from build123d import *

# Parameters (mm, degrees)
SKETCH1_W           = 50
SKETCH1_H           = 42
BOSS_EXTRUDE1_DEPTH = 16
SKETCH1_3_W         = 50
SKETCH1_3_H         = 42
BOSS_EXTRUDE2_DEPTH = 16
BOSS_EXTRUDE3_DEPTH = 35
BOSS_EXTRUDE4_DEPTH = 35
SKETCH3_R           = 10
BOSS_EXTRUDE5_DEPTH = 5


with BuildPart() as part:
    # Sketch1 → Boss-Extrude1 (new body)
    with BuildSketch(Plane.XY):
        Rectangle(SKETCH1_W, SKETCH1_H)
    extrude(amount=BOSS_EXTRUDE1_DEPTH)

    # Sketch1_3 → Boss-Extrude2 (add)
    with BuildSketch(Plane.XY):
        Rectangle(SKETCH1_3_W, SKETCH1_3_H)
    extrude(amount=-BOSS_EXTRUDE2_DEPTH)

    # Sketch1_4 → Boss-Extrude3 (add)
    with BuildSketch(Plane.XY):
        Polygon((-3, 28), (-3, 21), (25, 21), (34, 21), (34, 28), align=None)
    extrude(amount=BOSS_EXTRUDE3_DEPTH)

    # Sketch1_5 → Boss-Extrude4 (add)
    with BuildSketch(Plane.XY):
        Polygon((-3, 28), (-3, 21), (25, 21), (34, 21), (34, 28), align=None)
    extrude(amount=-BOSS_EXTRUDE4_DEPTH)

    # Sketch3 → Boss-Extrude5 (add)
    with BuildSketch(Plane.XZ.offset(21)):
        with Locations(Location((14, 0, 0), (0, 0, 90))):
            Circle(SKETCH3_R)
    extrude(amount=BOSS_EXTRUDE5_DEPTH)


solid = part.part
Input: part model. Units: mm. Frame: model coordinates. A direction names the side the tool comes from. Round coordinates to 2 decimals unless told otherwise and drop trailing zeros. Loops run counter-clockwise (first coordinate to the right, second up) from the corner with the lowest first, then second, coordinate; pieces in that order, holes last. Notation, with made-up numbers: (71, -31) -> (81, -31) arc R17 ccw to (81, -27) -> close; hole circle Ø2 at (20, -9). An arc over 180 degrees is marked (long way). Answer as a JSON object with one key per item and string values. Group by question number.
1) Ray query, L1, parallel to Y at x = -15.5, z = -13.5; L2, parallel to Z at x = -4, y = 9; L3, parallel to Y at x = 13, z = -20. Return the intervals inside material, ascending.
2) Section query B-B on z = 0. Output: boundary loops of the cut face in (x, y).
3) Section query A-A on x = 14. Output: boundary loops of the cut face in (y, z), plus the area to 3 significant figures.
4) Reachability of faces 1 (the flat face through (0, 0, -16)), 2 (the flat face through (-3, 25, 0)), 3 (the cylindrical face through (5.57, -23.46, 5.38)), 4 (the flat face through (0, 0, 16)) from +Z, -Z, +X, -X, +Y, -Y: full face, straight path, thin tool, end or side. Return the list, or none.
5) Pin query (flat end, axial travel): pin 1 (4 mm diameter, centred on x = 26, y = 3, fed in from +Z); pin 2 (12 mm diameter, centred on x = -5, y = -13, fed in from -Z); pin 3 (9.5 mm diameter, centred on y = -1, z = -4.5, fed in from +X). Return the tip coordinate at first contact, or that it passes through.
6) Section query C-C on y = -17. Output: boundary loops of the cut face in (x, z).
7) Section query D-D on z = -15. Output: boundary loops of the cut face in (x, y), plus the area to 3 significant figures.
Reply:
{
 "1": {"L1": "y = -21 to 21", "L2": "z = -16 to 16", "L3": "y = 21 to 28"},
 "2": {"outline": "(-25, -21) -> (4, -21) -> (4, -26) -> (24, -26) -> (24, -21) -> (25, -21) -> (25, 21) -> (34, 21) -> (34, 28) -> (-3, 28) -> (-3, 21) -> (-25, 21) -> close"},
 "3": {"outline": "(-26, -10) -> (-21, -10) -> (-21, -16) -> (21, -16) -> (21, -35) -> (28, -35) -> (28, 35) -> (21, 35) -> (21, 16) -> (-21, 16) -> (-21, 10) -> (-26, 10) -> close", "area": "1,930 mm2"},
 "4": {"face 1": "-Z, +X, -X, -Y", "face 2": "+Z, -Z, -X, +Y", "face 3": "-Y", "face 4": "+Z, +X, -X, -Y"},
 "5": {"pin 1": "stops at z = 16", "pin 2": "stops at z = -16", "pin 3": "stops at x = 25"},
 "6": {"outline": "(-25, -16) -> (25, -16) -> (25, 16) -> (-25, 16) -> close"},
 "7": {"outline": "(-25, -21) -> (25, -21) -> (25, 21) -> (34, 21) -> (34, 28) -> (-3, 28) -> (-3, 21) -> (-25, 21) -> close", "area": "2,360 mm2"}
}
